```python
from build123d import *

# Parameters (mm, degrees)
WALL_THICKNESS_T         = -3
FLANGE_PROFILE_W         = 216
FLANGE_PROFILE_H         = 216
FLANGE_PROFILE_W_2       = 153.219712456
FLANGE_PROFILE_H_2       = 152.670025112
MOUNTING_FLANGE_DEPTH    = 3
OUTLET_START             = 37
OUTLET_SIDE_FRONT_DEPTH  = 3
OUTLET_START_2           = -37
OUTLET_SIDE_REAR_DEPTH   = 3
OUTLET_BACK_DEPTH        = 40
SKETCH_6_R               = 2.5
JOINT_FIXING_HOLES_DEPTH = 40


with BuildPart() as part:
    # 草图1 → Hopper Shape section 0
    with BuildSketch(Plane(origin=(0, 0, 0), x_dir=(1, 0, 0), z_dir=(0, 1, 0))):
        with BuildLine():
            Line((-50, -40), (50, -40))
            Line((50, -40), (50, 40))
            Line((50, 40), (-50, 40))
            Line((-50, 40), (-50, -40))
        make_face()
    # Inlet Profile → Hopper Shape section 1
    with BuildSketch(Plane(origin=(0, 57, 0), x_dir=(1, 0, 0), z_dir=(0, 1, 0))):
        with BuildLine():
            Line((-80, -80), (80, -80))
            Line((80, -80), (80, 80))
            Line((80, 80), (-80, 80))
            Line((-80, 80), (-80, -80))
        make_face()
    loft()

    # Wall Thickness
    wall_thickness_openings = [part.faces().sort_by_distance(p)[0] for p in [
        (0, 57, 0),
        (0, 0, 0),
    ]]
    offset(amount=WALL_THICKNESS_T, openings=wall_thickness_openings, kind=Kind.INTERSECTION)

    # Flange Profile → Mounting Flange (add)
    with BuildSketch(Plane(origin=(0, 57, 0), x_dir=(1, 0, 0), z_dir=(0, 1, 0))):
        Rectangle(FLANGE_PROFILE_W, FLANGE_PROFILE_H)
        Rectangle(FLANGE_PROFILE_W_2, FLANGE_PROFILE_H_2, mode=Mode.SUBTRACT)
    extrude(amount=MOUNTING_FLANGE_DEPTH)

    # 草图3 → Outlet Side Front (add)
    with BuildSketch(Plane.XY.offset(OUTLET_START)):
        Polygon((-50, 0), (50, 0), (107.665544, -37.011165), (98.094598, -70.577127), (-50, -28.475092372), align=None)
    extrude(amount=OUTLET_SIDE_FRONT_DEPTH)

    # 草图4 → Outlet Side Rear (add)
    with BuildSketch(Plane.XY.offset(OUTLET_START_2)):
        Polygon((-50, 0), (50, 0), (107.665544, -37.011165), (98.094598, -70.577127), (-50, -28.475092372), align=None)
    extrude(amount=-OUTLET_SIDE_REAR_DEPTH)

    # 草图5 → Outlet Back (add, symmetric)
    with BuildSketch(Plane.XY):
        Polygon((-50, 0), (-47, 0), (-47, -29.327967372), (-50, -28.475092372), align=None)
    extrude(amount=OUTLET_BACK_DEPTH, both=True)

    # 草图6 → Joint Fixing Holes (cut, symmetric)
    with BuildSketch(Plane.XY):
        with Locations((93.124497189, -51.590532135)):
            Circle(SKETCH_6_R)
    extrude(amount=JOINT_FIXING_HOLES_DEPTH, both=True, mode=Mode.SUBTRACT)


solid = part.part
```
Geometry: final body of the model. Coordinates: model frame, mm. A direction names the side the tool comes from. Coordinates: 2 decimals unless noted, no trailing zeros. Write each loop counter-clockwise with the first axis right and the second up, starting at its lowest first coordinate (ties: lowest second). Pieces come first, ordered by that corner, then holes. Notation, with made-up numbers: M 74,77 L 88,77 A19 cw 88,89 Z; hole C 10,9 d10. An arc over 180 degrees is marked long. Answer as CSV lines item,"result". Start each with the question number.
Q1. Reachability of faces 5 (the flat face through (65.15, 35.23, 1.07)), 6 (the flat face through (30, -27, 40)), 7 (the flat face through (47, 0, -8)) from +Z, -Z, +X, -X, +Y, -Y: full face, straight path, thin tool, end or side. Return the list, or none.
Q2. Line query: line 1 (Z direction, x = 52, y = -56); line 2 (Y direction, x = 98, z = -10); line 3 (X direction, y = -8.5, z = -28). Output: solid intervals per line, ascending. Write a range as from..to.
Q3. Pin query (flat end, axial travel): P1, Ø21, axis at x = -0.5, y = -43.5, coming from the +Z side; P2, Ø1, axis at x = 58.5, z = -4.5, coming from the +Y side; P3, Ø14.5, axis at y = -18, z = -7.5, coming from the +X side. Return the tip coordinate at first contact, or that it passes through.
Q4. Cut plane B-B on z = 92. Return the cut outline in (x, y), then the cut area to 3 significant figures.
Q5. Cut plane D-D on x = -90. Return the cut outline in (y, z), then the cut area to 3 significant figures.
Q6. Cut plane A-A on y = -13.5. Return the cut outline in (x, z), then the cut area to 3 significant figures.
Q7. Cut plane C-C on y = -62.5. Return the cut outline in (x, z).
Q8. Mould query, pull axis X, two halves, no side actions, for faces 1 (the flat face through (31, -27, -37)), 2 (the flat face through (78.429, -18.247, -38.479)), 3 (the cylindrical face through (92.58, -54.03, -38.48)), 4 (the flat face through (-50, -14, 1)). Classes: released by +X, released by -X, zero draft, split by the parting line, or undercut.
Findings below:
1,face 5,"+Y"
1,face 6,"+Z, +X, -X, -Y"
1,face 7,"+X, -Y"
2,line 1,"z = -40..-37, 37..40"
2,line 2,"y = 57..60"
2,line 3,"x = -50..-47"
3,P1,"stops at z = 40"
3,P2,"stops at y = 23.54"
3,P3,"stops at x = -47"
4,outline,"M -108,57 L 108,57 L 108,60 L -108,60 Z"
4,area,"648 mm2"
5,outline,"M 57,-108 L 60,-108 L 60,108 L 57,108 Z"
5,area,"648 mm2"
6,outline,"M -50,-40 L 71.03,-40 L 71.03,-37 L -47,-37 L -47,37 L 71.03,37 L 71.03,40 L -50,40 Z"
6,area,"948 mm2"
7,outline,"M 69.68,-40 L 100.4,-40 L 100.4,-37 L 69.68,-37 Z; M 69.68,37 L 100.4,37 L 100.4,40 L 69.68,40 Z"
8,face 1,"zero draft"
8,face 2,"released by +X"
8,face 3,"undercut"
8,face 4,"released by -X"
